Can you work these out from the model? Positions are in its coordinate system, mm. Face numbers are marked on the shaded views. Coordinates: 2 decimals unless noted, no trailing zeros. Loops run counter-clockwise (first coordinate to the right, second up) from the corner with the lowest first, then second, coordinate; pieces in that order, holes last. Notation, with made-up numbers: (-37, 77.5) -> (6, 77.5) arc R19 ccw to (6, 104.5) -> close; hole circle Ø9 at (71.5, 2.25). An arc over 180 degrees is marked (long way). Use one line per item in the form item = value. Start each with the question number.
(1) I need wall thicknesses on line 1 (Y direction, x = 0, z = -4); line 2 (Y direction, x = 0, z = 14); line 3 (Z direction, x = 0, y = -20) (3 decimals). Which ranges of each line are inside material? Lowest first, please. Write a range as [from, to].
(2) Imagine slicing it at B-B (x = 0). List the corners of the cut face in (y, z) for me (3 decimals), plus the area to 3 significant figures.
(3) Thinking about a two-plate mould opening in X: for the marked faces 1, 2 and 3, which applies, released by +X, released by -X, zero draft, split by the parting line, or undercut?
(4) Imagine slicing it at A-A (z = 0). List the corners of the cut face in (x, y) for me (3 decimals), plus the area to 3 significant figures.
(5) Imagine slicing it at C-C (y = -38.1). List the corners of the cut face in (x, z) for me (3 decimals).
(6) Imagine slicing it at D-D (y = -7). List the corners of the cut face in (x, z) for me (3 decimals).
(7) I'm going to push flat-ended pins straight in: pin 1 (12 mm diameter, centred on y = -33, z = 2.5, fed in from -X) (3 decimals); pin 2 (6 mm diameter, centred on y = -34, z = -3.5, fed in from +X); pin 3 (10 mm diameter, centred on x = 2.5, y = -39, fed in from +Z); pin 4 (6 mm diameter, centred on y = -24.5, z = 6, fed in from -X). Where does each tip first touch, or does it pass through?
```python
from build123d import *

# Parameters (mm, degrees)
F0_R          = 15.875
F1_DEPTH      = 50.8
F4_R          = 2.54
F6_R          = 6.35
F7_DEPTH      = 15.875
F7_DEPTH_BACK = 15.875


with BuildPart() as f1:
    # F0 (on Front) → F1 (new body)
    with BuildSketch(Plane.XZ):
        Circle(F0_R)
    extrude(amount=F1_DEPTH)

    # F5: sweep along a path in F3
    with BuildLine(Plane(origin=(0, -12.7, 0), x_dir=(-1, 0, 0), z_dir=(0, 1, 0))) as f5_path:
        CenterArc((0, 0), 15.875, 0, 360)
    # F4 (on Right) → F5 (sweep, cut)
    with BuildSketch(Plane.YZ):
        with Locations((-12.7, 15.875)):
            Circle(F4_R)
    sweep(path=f5_path.line, mode=Mode.SUBTRACT)

    # F6 (on Top) → F7 (cut, two sides)
    with BuildSketch(Plane.XY) as f7_sk:
        with Locations((0, -38.1)):
            Circle(F6_R)
    extrude(amount=-F7_DEPTH, mode=Mode.SUBTRACT)
    extrude(f7_sk.sketch, amount=F7_DEPTH_BACK, mode=Mode.SUBTRACT)


solid = f1.part
```
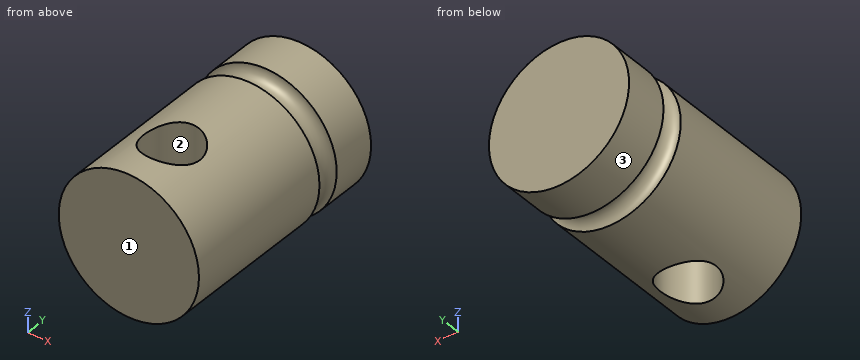
Worked out:
q1.line_1 = [-50.8, -44.45], [-31.75, 0]
q1.line_2 = [-50.8, -44.45], [-31.75, -14.41], [-10.99, 0]
q1.line_3 = [-15.875, 15.875]
q2.outline = (-50.8, -15.875) -> (-44.45, -15.875) -> (-44.45, 15.875) -> (-50.8, 15.875) -> close; (-31.75, -15.875) -> (-15.24, -15.875) arc R2.54 cw to (-10.16, -15.875) -> (0, -15.875) -> (0, 15.875) -> (-10.16, 15.875) arc R2.54 cw to (-15.24, 15.875) -> (-31.75, 15.875) -> close
q2.area = 1,190 mm2
q3.face_1 = zero draft
q3.face_2 = undercut
q3.face_3 = split by the parting line
q4.outline = (-15.875, -50.8) -> (15.875, -50.8) -> (15.875, -15.24) arc R2.54 cw to (15.875, -10.16) -> (15.875, 0) -> (-15.875, 0) -> (-15.875, -10.16) arc R2.54 cw to (-15.875, -15.24) -> close; hole circle Ø12.7 at (0, -38.1)
q4.area = 1,470 mm2
q5.outline = (-6.35, -14.55) -> (-6.35, 14.55) arc R15.875 ccw to start; (6.35, -14.55) arc R15.875 ccw to (6.35, 14.55) -> close
q6.outline = circle Ø31.75 at (0, 0)
q7.pin_1 = -15.875
q7.pin_2 = 15.87
q7.pin_3 = 15.7
q7.pin_4 = -15.59
